Check sheet for the modelled part. Datum: model origin and axes. Units: mm. Face numbers are marked on the shaded views. Give positions to 0.01 mm unless a question says otherwise; leave off trailing zeros. Loops run counter-clockwise (first coordinate to the right, second up) from the corner with the lowest first, then second, coordinate; pieces in that order, holes last. Notation, with made-up numbers: (-34, 57.25) - (-11, 57.25) arc R20 ccw to (-11, 61.25) - close; hole circle Ø7 at (34, -8). An arc over 180 degrees is marked (long way). Use CSV: the item, a comma, the result in double quotes.
from build123d import *

# Parameters (mm, degrees)
ESQUISSE1_R                  = 10
BOSS_EXTRU_1_DEPTH           = 40
ENL_V_MAT_EXTRU_1_DEPTH      = 95.339811321
ENL_V_MAT_EXTRU_2_DEPTH      = 95.339811321
ESQUISSE5_R                  = 3.075
ENL_V_MAT_EXTRU_3_DEPTH      = 50
ENL_V_MAT_EXTRU_4_DEPTH      = 95.339811321
TROU_TARAUD_M31_REACH        = 93.715
TROU_TARAUD_M31_BORE_R       = 1.25
BOSS_EXTRU_2_DEPTH           = 8
BOSS_EXTRU_3_DEPTH           = 8
ESQUISSE19_W                 = 7.5
ESQUISSE19_H                 = 30
ENL_V_MAT_EXTRU_5_DEPTH      = 1.5
BOSS_EXTRU_4_DEPTH           = 5
BOSS_EXTRU_5_DEPTH           = 5
ESQUISSE36_W                 = 50.627353798
ESQUISSE36_H                 = 3
BOSS_EXTRU_6_DEPTH           = 17
TROU_TARAUD_M35_D            = 2.5
TROU_TARAUD_M35_DEPTH        = 5
ESQUISSE40_R                 = 4.5
BOSS_EXTRU_8_DEPTH           = 5
ESQUISSE41_R                 = 3.075
ENL_V_MAT_EXTRU_7_DEPTH      = 5
ENL_V_MAT_EXTRU_8_DEPTH      = 101.831047543
ENL_V_MAT_EXTRU_8_DEPTH_BACK = 101.831047543
ESQUISSE42_R                 = 2.5


with BuildPart() as part:
    # Esquisse1 → Boss.-Extru.1 (new body)
    with BuildSketch(Plane(origin=(0, 0, 0), x_dir=(1, 0, 0), z_dir=(0, 1, 0))):
        with BuildLine():
            Line((0, -15), (80, -15))
            Line((80, -15), (80, 15))
            Line((80, 15), (0, 15))
            ThreePointArc((0, 15), (-15, 0), (0, -15))
        make_face()
        with Locations(Location((0, 0, 0), (0, 0, 270))):
            Circle(ESQUISSE1_R, mode=Mode.SUBTRACT)
    extrude(amount=BOSS_EXTRU_1_DEPTH)

    # Esquisse3 → Enlèv. mat.-Extru.1 (cut, through all)
    with BuildSketch(Plane.XY.offset(15)):
        Polygon((20, 0), (80, 0), (80, 21.8382), align=None)
    extrude(amount=-ENL_V_MAT_EXTRU_1_DEPTH, mode=Mode.SUBTRACT)

    # Esquisse4 → Enlèv. mat.-Extru.2 (cut, through all)
    with BuildSketch(Plane.XY.offset(15)):
        Polygon((80, 21.8382), (80, 40), (73.7889, 40), align=None)
    extrude(amount=-ENL_V_MAT_EXTRU_2_DEPTH, mode=Mode.SUBTRACT)

    # Esquisse5 → Enlèv. mat.-Extru.3 (cut)
    with BuildSketch(Plane(origin=(78.309664358, 26.780889355, 0), x_dir=(0, 0, -1), z_dir=(0.9461982424164683, 0.32358752455554646, 0))):
        with Locations(Location((0, 4.37351335, 0), (0, 0, 90))):
            Circle(ESQUISSE5_R)
    extrude(amount=-ENL_V_MAT_EXTRU_3_DEPTH, mode=Mode.SUBTRACT)

    # Esquisse6 → Enlèv. mat.-Extru.4 (cut, through all)
    with BuildSketch(Plane.XY.offset(15)):
        Polygon((75.083250098, 36.21520703), (20.083250098, 17.405920506), (12.356368008, 40), (73.7889, 40), align=None)
    extrude(amount=-ENL_V_MAT_EXTRU_4_DEPTH, mode=Mode.SUBTRACT)

    # Trou taraudé M31 bore → Trou taraudé M31 (cut, up to next)
    with BuildSketch(Plane(origin=(2.339552909, -6.427872928, 0), x_dir=(-0.9396926915369543, -0.3420199489387053, 0), z_dir=(0.3420199489387053, -0.9396926915369543, 0)), mode=Mode.PRIVATE) as trou_taraud_m31_sk1:
        with Locations((-46.885275043, 0)):
            Circle(TROU_TARAUD_M31_BORE_R)
    trou_taraud_m31_tool1 = extrude(trou_taraud_m31_sk1.sketch, amount=-TROU_TARAUD_M31_REACH, mode=Mode.PRIVATE) & part.part
    # Trou taraudé M31 bore → Trou taraudé M31 (cut, up to next)
    with BuildSketch(Plane(origin=(2.339552909, -6.427872928, 0), x_dir=(-0.9396926915369543, -0.3420199489387053, 0), z_dir=(0.3420199489387053, -0.9396926915369543, 0)), mode=Mode.PRIVATE) as trou_taraud_m31_sk2:
        with Locations((-70.089378087, 0)):
            Circle(TROU_TARAUD_M31_BORE_R)
    trou_taraud_m31_tool2 = extrude(trou_taraud_m31_sk2.sketch, amount=-TROU_TARAUD_M31_REACH, mode=Mode.PRIVATE) & part.part
    add(trou_taraud_m31_tool1.solids().sort_by_distance((46.397303, 9.607826, 0))[0], mode=Mode.SUBTRACT)
    add(trou_taraud_m31_tool2.solids().sort_by_distance((68.202029, 17.544093, 0))[0], mode=Mode.SUBTRACT)

    # Esquisse11 → Boss.-Extru.2 (add)
    with BuildSketch(Plane.XY.offset(15)):
        Polygon((20.083250098, 17.405920506), (16.847374853, 26.86790293), (12.116383641, 25.249965307), (15.352258886, 15.787982883), align=None)
    extrude(amount=BOSS_EXTRU_2_DEPTH)

    # Esquisse12 → Boss.-Extru.3 (add)
    with BuildSketch(Plane(origin=(0, 0, -15), x_dir=(-1, 0, 0), z_dir=(0, 0, -1))):
        Polygon((-20.083250098, 17.405920506), (-16.847374853, 26.86790293), (-12.116383641, 25.249965307), (-15.352258886, 15.787982883), align=None)
    extrude(amount=BOSS_EXTRU_3_DEPTH)

    # Esquisse19 → Enlèv. mat.-Extru.5 (cut)
    with BuildSketch(Plane(origin=(-3.22641426, 9.434317675, 0), x_dir=(0.9461982424164682, 0.3235875245555466, 0), z_dir=(-0.3235875245555466, 0.9461982424164682, 0))):
        with Locations((28.385074674, 0)):
            Rectangle(ESQUISSE19_W, ESQUISSE19_H)
    extrude(amount=-ENL_V_MAT_EXTRU_5_DEPTH, mode=Mode.SUBTRACT)

    # Esquisse34 → Boss.-Extru.4 (add)
    with BuildSketch(Plane.XY.offset(15)):
        Polygon((27.179736916, 19.83282694), (75.083250098, 36.21520703), (76.109211181, 33.21520703), (28.205697999, 16.83282694), align=None)
    extrude(amount=BOSS_EXTRU_4_DEPTH)

    # Esquisse35 → Boss.-Extru.5 (add)
    with BuildSketch(Plane(origin=(0, 0, -15), x_dir=(-1, 0, 0), z_dir=(0, 0, -1))):
        Polygon((-27.179736916, 19.83282694), (-75.083250098, 36.21520703), (-76.054012672, 33.376612303), (-28.15049949, 16.994232213), align=None)
    extrude(amount=BOSS_EXTRU_5_DEPTH)

    # Esquisse36 → Boss.-Extru.6 (add)
    with BuildSketch(Plane(origin=(-3.22641426, 9.434317675, 0), x_dir=(0.9461982424164682, 0.3235875245555466, 0), z_dir=(-0.3235875245555466, 0.9461982424164682, 0))):
        with Locations((57.448751573, -18.5)):
            Rectangle(ESQUISSE36_W, ESQUISSE36_H)
        with Locations((57.448751573, 18.5)):
            Rectangle(ESQUISSE36_W, ESQUISSE36_H)
    extrude(amount=BOSS_EXTRU_6_DEPTH)

    # Trou taraudé M35
    with Locations(Plane(origin=(23.309664358, 7.971602831, 0), x_dir=(0, 0, -1), z_dir=(0.9461982424164682, 0.3235875245555468, 0))):
        with Locations((-18.5, 14.970762206), (18.5, 14.970762206)):
            Hole(TROU_TARAUD_M35_D / 2, depth=TROU_TARAUD_M35_DEPTH)

    # Esquisse40 → Boss.-Extru.8 (add)
    with BuildSketch(Plane(origin=(78.309664358, 26.780889355, 0), x_dir=(0, 0, -1), z_dir=(0.9461982424164683, 0.32358752455554646, 0))):
        with Locations(Location((0, 4.37351335, 0), (0, 0, 270))):
            Circle(ESQUISSE40_R)
    extrude(amount=BOSS_EXTRU_8_DEPTH)

    # Esquisse41 → Enlèv. mat.-Extru.7 (cut)
    with BuildSketch(Plane(origin=(83.04065557, 28.398826978, 0), x_dir=(0, 0, -1), z_dir=(0.9461982424164683, 0.32358752455554646, 0))):
        with Locations(Location((0, 4.37351335, 0), (0, 0, 90))):
            Circle(ESQUISSE41_R)
    extrude(amount=-ENL_V_MAT_EXTRU_7_DEPTH, mode=Mode.SUBTRACT)

    # Esquisse42 → Enlèv. mat.-Extru.8 (cut, two sides: drawn at the far end of the back side and taken through both)
    with BuildSketch(Plane.XY.offset(-ENL_V_MAT_EXTRU_8_DEPTH_BACK)):
        with Locations(Location((0, 30, 0), (0, 0, 90.000000004))):
            Circle(ESQUISSE42_R)
        with Locations(Location((0, 10, 0), (0, 0, 90.000000004))):
            Circle(ESQUISSE42_R)
    extrude(amount=ENL_V_MAT_EXTRU_8_DEPTH + ENL_V_MAT_EXTRU_8_DEPTH_BACK, mode=Mode.SUBTRACT)


solid = part.part
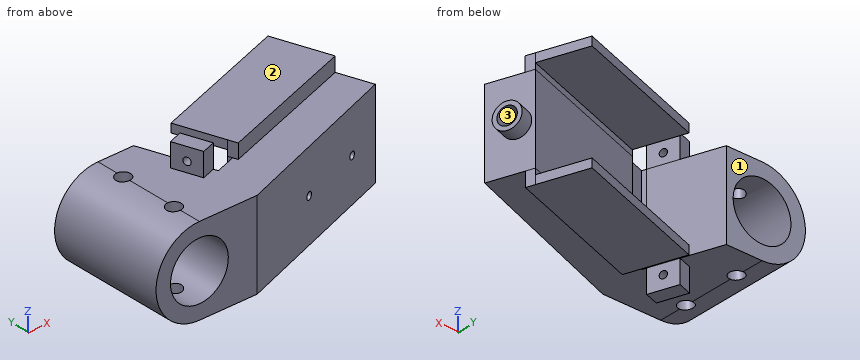
1. Sectioned sample at C-C, the plane z = 0. State how many separate pieces and enclosed holes the cut face has, and give its area (3 significant figures).
Completed:
separate pieces,"4"
enclosed holes,"0"
area,"1,140 mm²"
2. Sectioned sample at A-A, the plane y = 44.5. Record the boundary of the cut face in (x, z).
Completed:
outline,"(46.77, -20) - (72.25, -20) - (72.25, -17) - (46.77, -17) - close; (46.77, 17) - (72.25, 17) - (72.25, 20) - (46.77, 20) - close"
3. Sectioned sample at D-D, the plane y = 5.5. Record the boundary of the cut face in (x, z), and give its area (3 significant figures).
Completed:
outline,"(0, -15) - (35.11, -15) - (35.11, 15) - (0, 15) arc R15 ccw to start; hole circle Ø20 at (0, 0)"
area,"1,090 mm²"
4. Release check for a two-part mould opening along Y. For the marked faces 1, 2 and 3 record: released by +Y, released by -Y, zero draft, split by the parting line, or undercut.
Completed:
face 1,"released by +Y"
face 2,"zero draft"
face 3,"undercut"
5. Sectioned sample at B-B, the plane z = -12.5. Record the boundary of the cut face in (x, y), and give its area (3 significant figures).
Completed:
outline,"(-8.29, 0) - (20, 0) - (80, 21.84) - (75.08, 36.22) - (27.18, 19.83) - (27.67, 18.41) - (20.57, 15.99) - (12.36, 40) - (-8.29, 40) - close; hole circle Ø5 at (0, 10); hole circle Ø5 at (0, 30)"
area,"1,960 mm²"
6. Scan lines: line 1 along Y through (x, z) = (0, 13.55); line 2 along Z through (x, y) = (37.5, 31.5); line 3 along Z through (x, y) = (-9, 14.5). Record each from-to range of solid material in increasing order.
Completed:
line 1,"y = 0 to 7.5, 12.5 to 27.5, 32.5 to 40"
line 2,"z = -20 to -17, 17 to 20"
line 3,"z = -12 to -4.36, 4.36 to 12"
7. Go/stop test with flat-tipped pins: pin 1 Ø16 at (x, y) = (43, 31.5) entering from +Z; pin 2 Ø6 at (x, y) = (11.5, 36) entering from -Z; pin 3 Ø6 at (x, y) = (0, 10) entering from +Z; pin 4 Ø5 at (x, z) = (-0.5, -6) entering from +Y. Record where each tip stops, or that it passes through.
Completed:
pin 1,"stops at z = 20"
pin 2,"stops at z = -15"
pin 3,"stops at z = 15"
pin 4,"passes through"
